Can you work these out from the model? Positions are in its coordinate system, mm. Face numbers are marked on the shaded views. Give positions to 0.01 mm unless a question says otherwise; leave off trailing zeros. Write each loop counter-clockwise with the first axis right and the second up, starting at its lowest first coordinate (ties: lowest second). Pieces come first, ordered by that corner, then holes. Notation, with made-up numbers: (32.5, 83.5) -> (87.5, 83.5) arc R8 ccw to (87.5, 91.5) -> close; hole circle Ø8 at (18, -10). An arc over 180 degrees is marked (long way). Answer as CSV lines item,"result". Start each with the question number.
1. If we section it at D-D on z = 6: Write out the boundary of the cut face in (x, y).
2. If we section it at B-B on y = -35: Write out the boundary of the cut face in (x, z), plus the area to 3 significant figures.
3. If we mould it in two halves opening along X, with no side actions, what happens to the marked faces 1, 2 and 3? For each: pulls with the +X half, pulls with the -X half, needs draft (parallel to the pull), parting line crosses it, or undercut.
4. I need wall thicknesses on line 1 (X direction, y = -46, z = 6.5); line 2 (X direction, y = -42.5, z = 3.5); line 3 (Y direction, x = -49.5, z = 7.75). Which ranges of each line are inside material? Lowest first, please. Write a range as [from, to].
5. If we section it at A-A on x = 0: Write out the boundary of the cut face in (y, z).
6. I'm going to push flat-ended pins straight in: P1, Ø8, axis at y = 17, z = 2, coming from the +X side; P2, Ø22, axis at x = 42.67, y = 42.67, coming from the -Z side; P3, Ø2, axis at y = 38, z = 3, coming from the -X side; P4, Ø4, axis at y = -51, z = 11, coming from the +X side. Where does each tip first touch, or does it pass through?
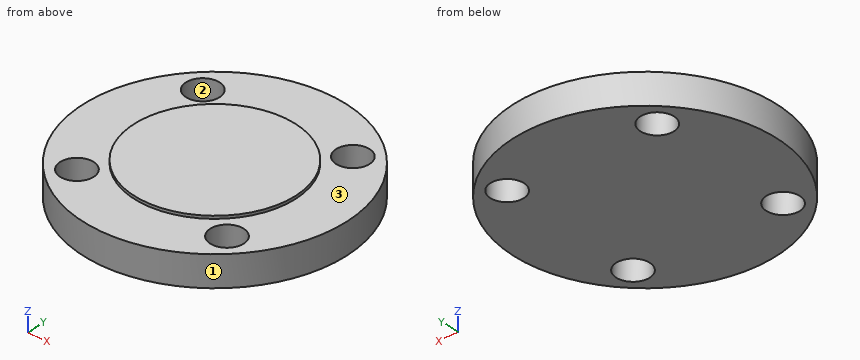
```python
from build123d import *

# Parameters (mm, degrees)
F2_R     = 75
F2_R_2   = 9.55
F2_R_3   = 45.95
F4_DEPTH = 17.5
F5_DEPTH = 19.1


with BuildPart() as f4:
    # F2 (on Top) → F4 (new body)
    with BuildSketch(Plane.XY):
        Circle(F2_R)
        with Locations((-42.6738942446, -42.6738942446)):
            Circle(F2_R_2, mode=Mode.SUBTRACT)
        with Locations((42.6738942446, -42.6738942446)):
            Circle(F2_R_2, mode=Mode.SUBTRACT)
        with Locations((-42.6738942446, 42.6738942446)):
            Circle(F2_R_2, mode=Mode.SUBTRACT)
        Circle(F2_R_3, mode=Mode.SUBTRACT)
        with Locations((42.6738942446, 42.6738942446)):
            Circle(F2_R_2, mode=Mode.SUBTRACT)
    extrude(amount=F4_DEPTH)

    # F2 (on Top) → F5 (join)
    with BuildSketch(Plane.XY):
        Circle(F2_R_3)
    extrude(amount=F5_DEPTH)


solid = f4.part
```
Computed values:
1,outline,"circle Ø150 at (0, 0); hole circle Ø19.1 at (-42.67, -42.67); hole circle Ø19.1 at (-42.67, 42.67); hole circle Ø19.1 at (42.67, -42.67); hole circle Ø19.1 at (42.67, 42.67)"
2,outline,"(-66.33, 0) -> (-48.36, 0) -> (-48.36, 17.5) -> (-66.33, 17.5) -> close; (-36.99, 0) -> (36.99, 0) -> (36.99, 17.5) -> (29.77, 17.5) -> (29.77, 19.1) -> (-29.77, 19.1) -> (-29.77, 17.5) -> (-36.99, 17.5) -> close; (48.36, 0) -> (66.33, 0) -> (66.33, 17.5) -> (48.36, 17.5) -> close"
2,area,"2,020 mm2"
3,face 1,"parting line crosses it"
3,face 2,"undercut"
3,face 3,"needs draft"
4,line 1,"x = [-59.24, -51.63], [-33.72, 33.72], [51.63, 59.24]"
4,line 2,"x = [-61.8, -52.22], [-33.13, 33.13], [52.22, 61.8]"
4,line 3,"y = [-56.34, -49.35], [-36, 36], [49.35, 56.34]"
5,outline,"(-75, 0) -> (75, 0) -> (75, 17.5) -> (45.95, 17.5) -> (45.95, 19.1) -> (-45.95, 19.1) -> (-45.95, 17.5) -> (-75, 17.5) -> close"
6,P1,"stops at x = 73.86"
6,P2,"stops at z = 0"
6,P3,"stops at x = -65.24"
6,P4,"stops at x = 56.78"
